The listing builds one solid part. Answer for the finished solid, in the listing's coordinates (mm). A direction names the side the tool comes from. Give positions to 0.01 mm unless a question says otherwise; leave off trailing zeros. Order: outer loops, then holes, each group sorted by start corner. A loop starts at its lowest first (then second) coordinate and runs counter-clockwise, first axis right, second up. Notation, with made-up numbers: (35.5, -5) - (66.5, -5) arc R21 cw to (66.5, 12) - close; hole circle Ø7 at (20.5, 32.5). An arc over 180 degrees is marked (long way). Answer in a Markdown table with one row per item. Add a question column.
```python
from build123d import *

# Parameters (mm, degrees)
F1_DEPTH    = 6.35
F2_DEPTH    = 25.4
F3_DEPTH    = 50.8
F4_R        = 6.34999
F5_SIZE     = 12.7
F6_C1_SIZE2 = 12.7
F6_C1_SIZE  = 7.3323484187
F6_C2_SIZE2 = 12.7
F6_C2_SIZE  = 7.3323484187
F6_C3_SIZE2 = 7.3323484187
F6_C3_SIZE  = 12.7
F6_C4_SIZE2 = 12.7
F6_C4_SIZE  = 7.3323484187


# Not quite as in the source:
# - a fillet or chamfer is up to 0.001 mm smaller than in the source, because OpenCascade refuses the exact size


with BuildPart() as f1:
    # F0 (on Top) → F1 (new body)
    with BuildSketch(Plane.XY):
        Polygon((-32.7964108223, 68.4432678408), (-121.6964108223, 68.7291226315), (-121.6964108223, -96.9018127685), (-32.7964108223, -96.6159616778), align=None)
        Polygon((-115.3464108223, 24.6241450903), (-115.3464108223, 62.3586716052), (-77.2464108223, 62.2361624092), (-39.1464108223, 62.1136532132), (-39.1464108223, -52.3088543971), (-39.1464108223, -90.2863467868), (-77.2464108223, -90.4088543971), (-115.3464108223, -90.5313620074), align=None, mode=Mode.SUBTRACT)
    extrude(amount=F1_DEPTH)

    # F0 (on Top) → F2 (join)
    with BuildSketch(Plane.XY):
        with BuildLine():
            Line((-90.1101133053, 24.2988232152), (-115.3464108223, 24.6241450903))
            Line((-115.3464108223, 24.6241450903), (-115.3464108223, -90.5313620074))
            Line((-115.3464108223, -90.5313620074), (-77.2464108223, -90.4088543971))
            Line((-77.2464108223, -90.4088543971), (-77.2464108223, -65.0088543971))
            ThreePointArc((-77.2464108223, -65.0088543971), (-73.5266669434, -56.028598276), (-64.5464108223, -52.3088543971))
            Line((-64.5464108223, -52.3088543971), (-39.1464108223, -52.3088543971))
            Line((-39.1464108223, -52.3088543971), (-39.1464108223, 62.1136532132))
            Line((-39.1464108223, 62.1136532132), (-77.2464108223, 62.2361624092))
            Line((-77.2464108223, 62.2361624092), (-77.2464108223, 36.9977681122))
            ThreePointArc((-77.2464108223, 36.9977681122), (-81.0242199909, 27.9598197407), (-90.1101133053, 24.2988232152))
        make_face()
    extrude(amount=F2_DEPTH)

    # F0 (on Top) → F3 (join)
    with BuildSketch(Plane.XY):
        with BuildLine():
            Line((-77.2464108223, -65.0088543971), (-77.2464108223, -90.4088543971))
            Line((-77.2464108223, -90.4088543971), (-39.1464108223, -90.2863467868))
            Line((-39.1464108223, -90.2863467868), (-39.1464108223, -52.3088543971))
            Line((-39.1464108223, -52.3088543971), (-64.5464108223, -52.3088543971))
            ThreePointArc((-64.5464108223, -52.3088543971), (-73.5266669434, -56.028598276), (-77.2464108223, -65.0088543971))
        make_face()
        with BuildLine():
            Line((-77.2464108223, 62.2361624092), (-115.3464108223, 62.3586716052))
            Line((-115.3464108223, 62.3586716052), (-115.3464108223, 24.6241450903))
            Line((-115.3464108223, 24.6241450903), (-90.1101133053, 24.2988232152))
            ThreePointArc((-90.1101133053, 24.2988232152), (-81.0242199909, 27.9598197407), (-77.2464108223, 36.9977681122))
            Line((-77.2464108223, 36.9977681122), (-77.2464108223, 62.2361624092))
        make_face()
    extrude(amount=F3_DEPTH)

    # F4 (radius 6.35 in the source; OpenCascade refuses exactly that, so slightly less here)
    f4_edges = [f1.edges().sort_by_distance(p)[0] for p in [
        (-77.246411, -96.758887, 6.35),
        (-32.796411, -14.086347, 6.35),
        (-77.246411, 68.586195, 6.35),
        (-121.696411, -14.086345, 6.35),
    ]]
    fillet(f4_edges, radius=F4_R)

    # F5
    f5_edges = [f1.edges().sort_by_distance(p)[0] for p in [
        (-96.296411, -90.470108, 25.4),
        (-39.146411, 4.902399, 25.4),
        (-115.346411, -32.953608, 25.4),
        (-58.196411, 62.174908, 25.4),
    ]]
    chamfer(f5_edges, length=F5_SIZE)

    # F6: chamfer of 12.7 x 7.3323484187 on 4 edges, made by hand

    # F6_c1
    f6_c1_edges = [f1.edges().sort_by_distance(p)[0] for p in [
        (-115.3464108223, 43.4914083477, 50.8),
    ]]
    f6_c1_side = f1.faces().sort_by_distance((-115.3464108223, 43.4914083477, 50.6533530316))[0]
    chamfer(f6_c1_edges, length=F6_C1_SIZE, length2=F6_C1_SIZE2, reference=f6_c1_side)

    # F6_c2
    f6_c2_edges = [f1.edges().sort_by_distance(p)[0] for p in [
        (-58.1964108223, -90.3476005919, 50.8),
    ]]
    f6_c2_side = f1.faces().sort_by_distance((-58.1964108223, -90.3476005919, 50.6533530316))[0]
    chamfer(f6_c2_edges, length=F6_C2_SIZE, length2=F6_C2_SIZE2, reference=f6_c2_side)

    # F6_c3
    f6_c3_edges = [f1.edges().sort_by_distance(p)[0] for p in [
        (-89.9464108223, 62.2769988079, 50.8),
    ]]
    f6_c3_side = f1.faces().sort_by_distance((-89.9464108223, 62.2769988079, 50.6533530316))[0]
    chamfer(f6_c3_edges, length=F6_C3_SIZE, length2=F6_C3_SIZE2, reference=f6_c3_side)

    # F6_c4
    f6_c4_edges = [f1.edges().sort_by_distance(p)[0] for p in [
        (-39.1464108223, -64.9475677659, 50.8),
    ]]
    f6_c4_side = f1.faces().sort_by_distance((-39.1464108223, -64.9475677659, 50.6533530316))[0]
    chamfer(f6_c4_edges, length=F6_C4_SIZE, length2=F6_C4_SIZE2, reference=f6_c4_side)


solid = f1.part
```
(1) The mould has two halves that part along Y. Classify faces 4 (the face through (-77.87, 66.68, 4.54)), 5 (the face through (-39.146, -49, 12)), 6 (the face through (-76.63, -94.847, 4.539)): +Y half, -Y half, draft (parallel to the pull), parting line (faces both ways), or undercut.
(2) Straight lines are drawn through the part: line 1 (X direction, y = 40.5, z = 39); line 2 (X direction, y = -81.5, z = 11.5); line 3 (Z direction, x = -52, y = -20). For each, find the intervals that lie inside material, in ascending order.
(3) Find section A-A, the plane z = 28.5. Write down the section's boundary in (x, y).
(4) For faces 1 (the face through (-45.585, 4.101, 19.139)), 2 (the face through (-119.787, -15.246, 4.539)), 3 (the face through (-108.908, -32.148, 19.139)), determine the directions among +Z, -Z, +X, -X, +Y, -Y from which every point of the face is accessible in a straight line to the end or side of a thin tool.
(5) Each of these flat-tipped pins is pushed along its axis until it touches: P1, Ø6, axis at x = -105, z = 24, coming from the +Y side; P2, Ø8, axis at x = -64, y = -16.5, coming from the +Z side; P3, Ø2, axis at y = 15, z = 17.5, coming from the -X side. Where does it stop, or does it pass through?
(6) Find section D-D, the plane z = 9. Write down the section's boundary in (x, y), plus the area to 3 significant figures.
(7) Find section C-C, the plane z = 48.5. Write down the section's boundary in (x, y), plus the area to 3 significant figures.
Answer key:
| question | item | result |
|---|---|---|
| 1 | face 4 | +Y half |
| 1 | face 5 | draft |
| 1 | face 6 | -Y half |
| 2 | line 1 | -115.35 to -77.25 |
| 2 | line 2 | -115.35 to -39.15 |
| 2 | line 3 | 0 to 25.4 |
| 3 | outline | (-115.35, 24.62) - (-90.11, 24.3) arc R12.7 ccw to (-77.25, 37) - (-77.25, 62.24) - (-115.35, 62.36) - close; (-77.25, -90.41) - (-39.15, -90.29) - (-39.15, -52.31) - (-64.55, -52.31) arc R12.7 ccw to (-77.25, -65.01) - close |
| 4 | face 1 | +Z, +X, +Y |
| 4 | face 2 | +Z, -X, +Y, -Y |
| 4 | face 3 | +Z, -X, -Y |
| 5 | P1 | y = 62.34 |
| 5 | P2 | z = 25.4 |
| 5 | P3 | x = -111.55 |
| 6 | outline | (-115.35, -90.53) - (-39.15, -90.29) - (-39.15, 62.11) - (-115.35, 62.36) - close |
| 6 | area | 11,600 mm² |
| 7 | outline | (-106.63, 24.51) - (-90.11, 24.3) arc R12.7 ccw to (-77.25, 37) - (-77.25, 56.23) - (-106.63, 56.33) - close; (-77.25, -81.69) - (-47.86, -81.6) - (-47.86, -52.31) - (-64.55, -52.31) arc R12.7 ccw to (-77.25, -65.01) - close |
| 7 | area | 1,730 mm² |
